```python
from build123d import *

# Parameters (mm, degrees)
SKETCH2_W           = 98
SKETCH2_H           = 42
BOSS_EXTRUDE1_DEPTH = 10
SKETCH3_W           = 64.32909673
SKETCH3_H           = 10
CUT_EXTRUDE3_DEPTH  = 108.088748242
SKETCH4_W           = 42
SKETCH4_H           = 42
BOSS_EXTRUDE2_DEPTH = 7
FILLET1_R           = 21
SKETCH5_R           = 10
CUT_EXTRUDE4_DEPTH  = 14
SKETCH7_R           = 6
CUT_EXTRUDE6_DEPTH  = 115.594938806
FILLET5_R           = 5
FILLET6_R           = 5
FILLET7_R           = 5


with BuildPart() as part:
    # Sketch2 → Boss-Extrude1 (new, symmetric)
    with BuildSketch(Plane(origin=(0, 0, 0), x_dir=(1, 0, 0), z_dir=(0, 1, 0))):
        with Locations((49, 21)):
            Rectangle(SKETCH2_W, SKETCH2_H)
    extrude(amount=BOSS_EXTRUDE1_DEPTH, both=True)

    # Sketch3 → Cut-Extrude3 (cut, through all)
    with BuildSketch(Plane.XY):
        with Locations((44.363668704, -5)):
            Rectangle(SKETCH3_W, SKETCH3_H)
    extrude(amount=-CUT_EXTRUDE3_DEPTH, mode=Mode.SUBTRACT)

    # Sketch4 → Boss-Extrude2 (add, symmetric)
    with BuildSketch(Plane(origin=(49, 0, 0), x_dir=(0, 0, -1), z_dir=(1, 0, 0))):
        with Locations((21, 31)):
            Rectangle(SKETCH4_W, SKETCH4_H)
    extrude(amount=BOSS_EXTRUDE2_DEPTH, both=True)

    # Fillet1
    fillet1_edges = [part.edges().sort_by_distance(p)[0] for p in [
        (49, 52, 0),
        (49, 52, -42),
    ]]
    fillet(fillet1_edges, radius=FILLET1_R - 0.0001)  # a hair under: the kernel refuses the full size

    # Sketch5 → Cut-Extrude4 (cut)
    with BuildSketch(Plane(origin=(56, 0, 0), x_dir=(0, 0, -1), z_dir=(1, 0, 0))):
        with Locations((21, 31)):
            Circle(SKETCH5_R)
    extrude(amount=-CUT_EXTRUDE4_DEPTH, mode=Mode.SUBTRACT)

    # Sketch7 → Cut-Extrude6 (cut, through all)
    with BuildSketch(Plane(origin=(0, 10, 0), x_dir=(1, 0, 0), z_dir=(0, 1, 0))):
        with Locations(Location((24, 21, 0), (0, 0, 270))):
            Circle(SKETCH7_R)
    cut_extrude6 = extrude(amount=-CUT_EXTRUDE6_DEPTH, mode=Mode.SUBTRACT)

    # Mirror3: Cut-Extrude6 across plane
    add(cut_extrude6.mirror(Plane(origin=(49, 0, 0), x_dir=(0, 0, 1), z_dir=(1, 0, 0))), mode=Mode.SUBTRACT)

    # Fillet5
    fillet5_edges = [part.edges().sort_by_distance(p)[0] for p in [
        (98, 10, -21),
    ]]
    fillet(fillet5_edges, radius=FILLET5_R)

    # Fillet6
    fillet6_edges = [part.edges().sort_by_distance(p)[0] for p in [
        (0, 10, -21),
    ]]
    fillet(fillet6_edges, radius=FILLET6_R)

    # Fillet7
    fillet7_edges = [part.edges().sort_by_distance(p)[0] for p in [
        (42, 10, -21),
        (56, 10, -21),
    ]]
    fillet(fillet7_edges, radius=FILLET7_R)


solid = part.part
```
CAD build for the part. Positions are in the model's coordinates, mm. A direction names the side the tool comes from. Give positions to 0.01 mm unless a question says otherwise; leave off trailing zeros. Order: outer loops, then holes, each group sorted by start corner. A loop starts at its lowest first (then second) coordinate and runs counter-clockwise, first axis right, second up.
(1) Saw through at C-C, the plane z = -29. Give the cut face in (x, y), then the cut area to 3 significant figures.
(2) Mould opens along X. For faces 1 (the flat face through (0, -2, -21)), 2 (the cylindrical face through (49.098, 22.128, -25.614)), 3 (the cylindrical face through (79.857, 2.362, -22.301)), 4 (the flat face through (12.199, -5, -21)) say: released by +X, released by -X, zero draft, split by the parting line, or undercut.
(3) Saw through at D-D, the plane z = -19.5. Give the cut face in (x, y).
(4) Saw through at A-A, the plane x = 74. Give the cut face in (y, z).
(5) Saw through at B-B, the plane y = -1. Give the cut face in (x, z), then the cut area to 3 significant figures.
(6) Flat gauge pins, fed straight in: pin 1 (12.5 mm diameter, centred on x = 28.5, z = -31, fed in from -Y); pin 2 (1 mm diameter, centred on y = 26.5, z = -4.5, fed in from +X); pin 3 (3 mm diameter, centred on y = 7, z = -14.5, fed in from +X). Where does each tip first touch, or does it go through?
(7) Drill centre lines: L1, parallel to X at y = 2.75, z = -21; L2, parallel to X at y = -1, z = -21; L3, parallel to X at y = -4, z = -9. Where is each one in solid material? Low to high.
(8) Tool access for faces 5 (the cylindrical face through (48.902, 45.685, -5.988)), 6 (the flat face through (56, 34, -11)), 7 (the flat face through (17, 10, -21)), 8 (the flat face through (76.528, -5, -8)): list every direction of +Z, -Z, +X, -X, +Y, -Y with a clear straight run to the whole face (end or side of a thin tool).
Results found:
1. outline: (0, -10) - (12.2, -10) - (12.2, 0) - (76.53, 0) - (76.53, -10) - (98, -10) - (98, 5) arc R5 ccw to (93, 10) - (61, 10) arc R5 cw to (56, 15) - (56, 25) - (42, 25) - (42, 15) arc R5 cw to (37, 10) - (5, 10) arc R5 ccw to (0, 5) - close; (42, 37) - (56, 37) - (56, 50.42) - (42, 50.42) - close
1. area: 1,710 mm2
2. face 1: released by -X
2. face 2: zero draft
2. face 3: undercut
2. face 4: undercut
3. outline: (0, -10) - (12.2, -10) - (12.2, 0) - (18.19, 0) - (18.19, 10) - (5, 10) arc R5 ccw to (0, 5) - close; (29.81, 0) - (68.19, 0) - (68.19, 10) - (61, 10) arc R5 cw to (56, 15) - (56, 21.11) - (42, 21.11) - (42, 15) arc R5 cw to (37, 10) - (29.81, 10) - close; (42, 40.89) - (56, 40.89) - (56, 51.95) - (42, 51.95) - close; (79.81, -10) - (98, -10) - (98, 5) arc R5 ccw to (93, 10) - (79.81, 10) - close
4. outline: (0, -42) - (10, -42) - (10, -27) - (0, -27) - close; (0, -15) - (10, -15) - (10, 0) - (0, 0) - close
5. outline: (0, -42) - (12.2, -42) - (12.2, 0) - (0, 0) - close; (76.53, -42) - (98, -42) - (98, 0) - (76.53, 0) - (76.53, -15.56) arc R6 cw to (76.53, -26.44) - close
5. area: 1,390 mm2
6. pin 1: stops at y = 0
6. pin 2: stops at x = 56
6. pin 3: stops at x = 97.97
7. L1: x = 0 to 18, 30 to 68, 80 to 98
7. L2: x = 0 to 12.2, 80 to 98
7. L3: x = 0 to 12.2, 76.53 to 98
8. face 5: +Z, +X, -X, +Y
8. face 6: +Z, -Z, +X, +Y
8. face 7: +Z, -Z, -X, +Y
8. face 8: +Z, -Z, -Y
